Verification items for the finished model (mm, model axes). Coordinates: 2 decimals unless noted, no trailing zeros. Order: outer loops, then holes, each group sorted by start corner. A loop starts at its lowest first (then second) coordinate and runs counter-clockwise, first axis right, second up. Notation, with made-up numbers: (-35.75, -21.75) - (-7.75, -21.75) arc R31 ccw to (-7.75, 12.25) - close; hole circle Ø2 at (79.25, -32). An arc over 180 degrees is marked (long way). Answer as CSV lines item,"result". Start each with the question number.
1. Section check C-C (y = 100). Record the cut outline in (x, z).
2. Section check A-A (x = 2.9). Record the cut outline in (y, z), and give its area (4 significant figures).
3. Material ranges on L1, parallel to Z at x = 1, y = 23; L2, parallel to Z at x = 4.5, y = 111.5; L3, parallel to Y at x = 2.4, z = -80, recorded low to high. Write a range as [from, to].
4. Go/stop test with flat-tipped pins: pin 1 (1.5 mm diameter, centred on x = 3.5, y = 152.5, fed in from -Z); pin 2 (2.5 mm diameter, centred on x = 2.5, z = -183.5, fed in from -Y); pin 3 (1.5 mm diameter, centred on x = 3.5, y = -4.5, fed in from +Z). Record where each tip stops, or that it passes through.
5. Section check D-D (z = -154). Record the cut outline in (x, y).
6. Section check B-B (z = -108). Record the cut outline in (x, y).
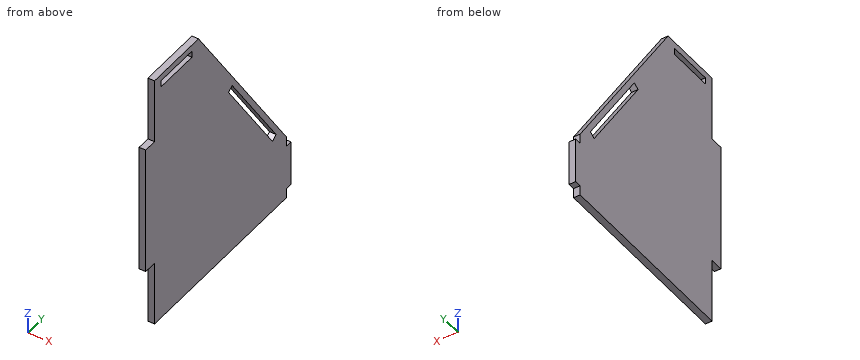
from build123d import *

# Parameters (mm, degrees)
CROQUIS1_W              = 5
CROQUIS1_H              = 35
SALIENTE_EXTRUIR1_DEPTH = 5


with BuildPart() as part:
    # Croquis1 → Saliente-Extruir1 (new body)
    with BuildSketch(Plane(origin=(0, 0, 0), x_dir=(0, 0, -1), z_dir=(1, 0, 0))):
        Polygon((150, 150), (0, 50), (0, 0), (50, 0), (50, -10), (150, -10), (150, 0), (200, 0), (200, 150), (192.5, 150), (192.5, 155), (157.5, 155), (157.5, 150), align=None)
        with Locations((7.5, 25)):
            Rectangle(CROQUIS1_W, CROQUIS1_H, mode=Mode.SUBTRACT)
        Polygon((65, 88.333333333), (139.88452649, 138.256350994), (142.658027472, 134.096099522), (67.773500981, 84.173081862), align=None, mode=Mode.SUBTRACT)
    extrude(amount=SALIENTE_EXTRUIR1_DEPTH)


solid = part.part
Evaluation:
1,outline,"(0, -200) - (5, -200) - (5, -91.51) - (0, -91.51) - close; (0, -82.5) - (5, -82.5) - (5, -75) - (0, -75) - close"
2,outline,"(-10, -150) - (0, -150) - (0, -200) - (150, -200) - (150, -192.5) - (155, -192.5) - (155, -157.5) - (150, -157.5) - (150, -150) - (50, 0) - (0, 0) - (0, -50) - (-10, -50) - close; hole (7.5, -10) - (42.5, -10) - (42.5, -5) - (7.5, -5) - close; hole (84.17, -67.77) - (134.1, -142.66) - (138.26, -139.88) - (88.33, -65) - close"
2,area,"23,050 mm²"
3,L1,"z = [-200, -10], [-5, 0]"
3,L2,"z = [-200, -108.76], [-99.75, -92.25]"
3,L3,"y = [-10, 92.32], [98.33, 103.33]"
4,pin 1,"stops at z = -192.5"
4,pin 2,"stops at y = 0"
4,pin 3,"stops at z = -50"
5,outline,"(0, 0) - (5, 0) - (5, 150) - (0, 150) - close"
6,outline,"(0, -10) - (5, -10) - (5, 110.99) - (0, 110.99) - close; (0, 117) - (5, 117) - (5, 122) - (0, 122) - close"
